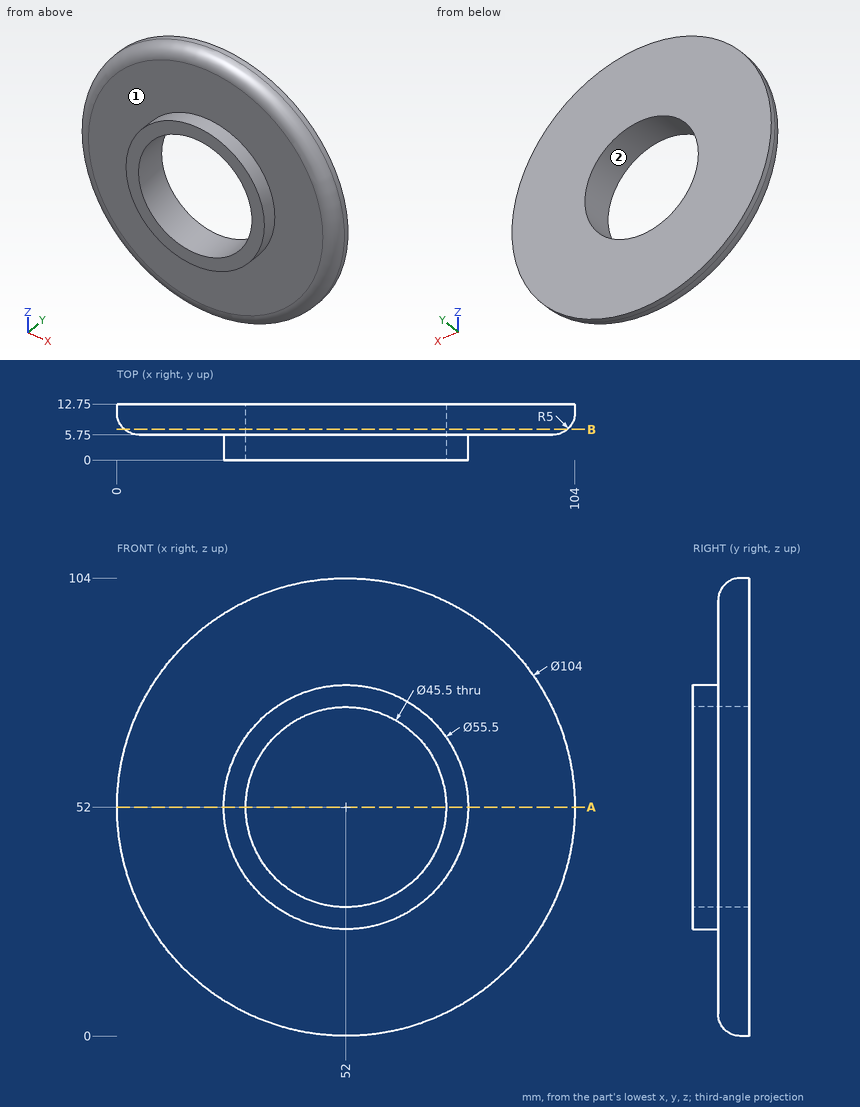
Source: three-view drawing plus pictorial views. Frame: mm from the lowest corner of the part. Give positions to 0.01 mm unless a question says otherwise; leave off trailing zeros. Order: outer loops, then holes, each group sorted by start corner. A loop starts at its lowest first (then second) coordinate and runs counter-clockwise, first axis right, second up. Notation, with made-up numbers: M 16,24.25 L 54,24.25 A13 cw 54,41.25 Z; hole C 20,-7 d1. An arc over 180 degrees is marked long. Return JSON: item names as keys, results as strings.
Item 1: First-contact query: P1, Ø5, axis at x = 43, y = 2.5, coming from the -Z side; P2, Ø1.5, axis at y = 7.5, z = 72.5, coming from the +X side; P3, Ø5, axis at x = 37.5, y = 7, coming from the -Z side. Flat tips, straight axial feed; report the tip coordinate or a pass-through.
Solutions:
{"P1": "z = 25.02", "P2": "x = 99.16", "P3": "z = 1.98"}
Item 2: Ray query, probe 1 along Z at (x, y) = (52, 3.5); probe 2 along Y at (x, z) = (58, 98); probe 3 along X at (y, z) = (12, 67). Return the intervals inside material, ascending.
Solutions:
{"probe 1": "24.25 to 29.25, 74.75 to 79.75", "probe 2": "5.75 to 12.75", "probe 3": "2.21 to 34.9, 69.1 to 101.79"}
Item 3: Cut plane B-B (y = 7). Return loops of the section in (x, z), then the cut area to 3 significant figures.
Solutions:
{"outline": "C 52,52 d100.61; hole C 52,52 d45.5", "area": "6,320 mm^2"}
Item 4: Cut plane A-A (z = 52). Return loops of the section in (x, y), then the cut area to 3 significant figures.
Solutions:
{"outline": "M 0,10.75 A5 ccw 5,5.75 L 24.25,5.75 L 24.25,0 L 29.25,0 L 29.25,12.75 L 0,12.75 Z; M 74.75,0 L 79.75,0 L 79.75,5.75 L 99,5.75 A5 ccw 104,10.75 L 104,12.75 L 74.75,12.75 Z", "area": "456 mm^2"}
Item 5: Pull-direction query (X, two-part tool) for the marked faces 1 and 2; classes: +X half, -X half, draft (parallel to the pull), parting line (faces both ways), or undercut.
Solutions:
{"face 1": "draft", "face 2": "undercut"}
